CAD build for the part. Positions are in the model's coordinates, mm. A direction names the side the tool comes from. Round coordinates to 2 decimals unless told otherwise and drop trailing zeros. Write each loop counter-clockwise with the first axis right and the second up, starting at its lowest first coordinate (ties: lowest second). Pieces come first, ordered by that corner, then holes. Notation, with made-up numbers: (36.5, -1.75) -> (75.5, -1.75) arc R4 ccw to (75.5, 5.25) -> close; hole circle Ø1 at (38, 60). An arc over 180 degrees is marked (long way). Put each result on its own line as item: value. Start each with the question number.
1. Saw through at C-C on y = 35. List the corners of the cut face in (x, z).
2. Saw through at B-B on y = 16. List the corners of the cut face in (x, z).
3. Flat gauge pins, fed straight in: P1, Ø1, axis at y = 20, z = -0.5, coming from the -X side; P2, Ø1, axis at x = -5.5, z = 0.5, coming from the +Y side; P3, Ø0.8, axis at x = -6.5, y = 32.5, coming from the +Z side. Where does each tip first touch, or does it go through?
4. 3-axis set-ups, long thin cutter, end or side, ignore diameter. For faces 1 (the cylindrical face through (-4.3, 34.6, 0.3)), 2 (the cylindrical face through (-3.674, -0.626, 0.683)): which of +Z, -Z, +X, -X, +Y, -Y reach the whole face in a straight line?
5. Saw through at A-A on z = 0.8. List the corners of the cut face in (x, y), and give its area (3 significant figures).
6. Drill centre lines: line 1 (Y direction, x = -6.15, z = 0.3); line 2 (Y direction, x = -6.95, z = 1.25); line 3 (Z direction, x = -5.5, y = 10.5). Where is each one in solid material? Low to high. Write a range as from..to.
7. Pull direction Y, two halves, no side cores. Call faces 3 (the flat face through (-6, 36.068, 0)), 4 (the flat face through (-6, -1.27, 0)), 5 (the cylindrical face through (-4.831, 15.233, 0.054)), 6 (the cylindrical face through (-6.465, 37.098, 0.904)): pulls with the +Y half, pulls with the -Y half, needs draft (parallel to the pull), parting line crosses it, or undercut.
from build123d import *

# Parameters (mm, degrees)
SKETCH1_R           = 0.8255
BOSS_EXTRUDE1_DEPTH = 38.1
SKETCH3_R           = 1.905
BOSS_EXTRUDE2_DEPTH = 1.27
SKETCH6_R           = 1.27
BOSS_EXTRUDE5_DEPTH = 7.200607359
SKETCH8_R           = 1.016
CUT_EXTRUDE2_DEPTH  = 2.032
SKETCH9_W           = 0.40474265
SKETCH9_H           = 1.016
CUT_EXTRUDE3_DEPTH  = 0.762


with BuildPart() as part:
    # Sketch1 → Boss-Extrude1 (new body)
    with BuildSketch(Plane(origin=(0, 0, 0), x_dir=(1, 0, 0), z_dir=(0, 1, 0))):
        with Locations(Location((-5.56320867, -0.435127994, 0), (0, 0, 90))):
            Circle(SKETCH1_R)
    extrude(amount=BOSS_EXTRUDE1_DEPTH)

    # Sketch3 → Boss-Extrude2 (add)
    with BuildSketch(Plane.XZ):
        with Locations(Location((-5.56320867, 0.435127994, 0), (0, 0, 270))):
            Circle(SKETCH3_R)
    extrude(amount=BOSS_EXTRUDE2_DEPTH)

    # Sketch6 → Boss-Extrude5 (add)
    with BuildSketch(Plane(origin=(0, 38.1, 0), x_dir=(1, 0, 0), z_dir=(0, 1, 0))):
        with Locations(Location((-5.56320867, -0.435127994, 0), (0, 0, 270))):
            Circle(SKETCH6_R)
    extrude(amount=-BOSS_EXTRUDE5_DEPTH)

    # Sketch8 → Cut-Extrude2 (cut)
    with BuildSketch(Plane(origin=(0, 38.1, 0), x_dir=(1, 0, 0), z_dir=(0, 1, 0))):
        with Locations(Location((-5.56320867, -0.435127994, 0), (0, 0, 270))):
            Circle(SKETCH8_R)
    extrude(amount=-CUT_EXTRUDE2_DEPTH, mode=Mode.SUBTRACT)

    # Sketch9 → Cut-Extrude3 (cut)
    with BuildSketch(Plane.ZY.offset(6.83320867)):
        with Locations((0.202371325, 32.386805083)):
            Rectangle(SKETCH9_W, SKETCH9_H)
    extrude(amount=-CUT_EXTRUDE3_DEPTH, mode=Mode.SUBTRACT)


solid = part.part
Return value:
1. outline: circle Ø2.54 at (-5.56, 0.44)
2. outline: circle Ø1.65 at (-5.56, 0.44)
3. P1: stops at x = -6.26
3. P2: stops at y = 36.07
3. P3: stops at z = 1.59
4. face 1: +Y
4. face 2: +Y, -Y
5. outline: (-7.43, -1.27) -> (-3.69, -1.27) -> (-3.69, 0) -> (-4.82, 0) -> (-4.82, 30.9) -> (-4.35, 30.9) -> (-4.35, 38.1) -> (-4.61, 38.1) -> (-4.61, 36.07) -> (-6.51, 36.07) -> (-6.51, 38.1) -> (-6.78, 38.1) -> (-6.78, 30.9) -> (-6.3, 30.9) -> (-6.3, 0) -> (-7.43, 0) -> close
5. area: 64.2 mm^2
6. line 1: y = -1.27..31.88, 32.89..36.07
6. line 2: y = -1.27..0
6. line 3: z = -0.39..1.26
7. face 3: pulls with the +Y half
7. face 4: pulls with the -Y half
7. face 5: undercut
7. face 6: needs draft
